from build123d import *

# Parameters (mm, degrees)
F0_W      = 1284.835703671
F0_H      = 12.4089680612
F1_DEPTH  = 571.5
F3_DEPTH  = 1143
F6_W      = 51.6073703766
F6_H      = 47.9507148266
F7_DEPTH  = 1778
F8_W      = 51.4650344849
F8_H      = 51.4650344849
F9_DEPTH  = 508
F10_W     = 63.6484324932
F10_H     = 50.9061813354
F10_W_2   = 66.0638809204
F10_H_2   = 51.4912605286
F11_DEPTH = 1092.2
F12_W     = 1241.9298887253
F12_H     = 1109.2171669006
F13_DEPTH = 139.7
F14_W     = 296.2205260992
F14_H     = 70.9949955344
F14_W_2   = 408.8332653046
F14_H_2   = 83.2355730236
F15_DEPTH = 1127.2688971291
F16_W     = 894.5828676224
F16_H     = 889.6675109863
F17_DEPTH = 1320.8


with BuildPart() as f1:
    # F0 (on Front) → F1 (new body, symmetric)
    with BuildSketch(Plane.XZ):
        with Locations((576.5165500343, -47.0742117614)):
            Rectangle(F0_W, F0_H)
    extrude(amount=F1_DEPTH, both=True)

    # F2 (on face) → F3 (join)
    with BuildSketch(Plane.XZ.offset(571.5)):
        Polygon((-65.9013018012, -53.278695792), (-65.9013018012, -40.8697277308), (-65.9013018012, 93.3853983879), (-249.7984468937, 93.3853983879), (-249.7984468937, 77.8451710939), (-80.1585838199, 77.8451710939), (-80.1585838199, -53.278695792), align=None)
    extrude(amount=-F3_DEPTH)

    # F5: F1 across plane


with BuildPart() as f1_1:
    add(f1.part)
    add(f1.part.mirror(Plane(origin=(569.387909025, 0, -17.3954870552), x_dir=(0, -1, 0), z_dir=(-1, 0, 0))))

    # F6 (on face) → F7 (join)
    with BuildSketch(Plane.XY.offset(-40.8697277308)):
        with Locations((569.3829655647, 546.9712764025)):
            Rectangle(F6_W, F6_H)
    extrude(amount=F7_DEPTH)

    # F8 (on mid) → F9 (join, symmetric)
    with BuildSketch(Plane(origin=(569.387909025, 0, 0), x_dir=(0, -1, 0), z_dir=(-1, 0, 0))):
        with Locations((-546.9267964363, 1710.9147310257)):
            Rectangle(F8_W, F8_H)
    extrude(amount=F9_DEPTH, both=True)

    # F10 (on face) → F11 (join)
    with BuildSketch(Plane.XZ.offset(-521.1942791939)):
        with Locations((93.3082550764, 1711.1941576004)):
            Rectangle(F10_W, F10_H)
        with Locations((1043.2767868042, 1710.7145786285)):
            Rectangle(F10_W_2, F10_H_2)
    extrude(amount=F11_DEPTH)

    # F12 (on face) → F13 (join)
    with BuildSketch(Plane.XY.offset(-40.8697277308)):
        with Locations((564.4726157188, 0)):
            Rectangle(F12_W, F12_H)
    extrude(amount=F13_DEPTH)

    # F14 (on face) → F15 (cut, through all)
    with BuildSketch(Plane.XZ.offset(554.6085834503)):
        with Locations((122.6859763265, 33.3608575165)):
            Rectangle(F14_W, F14_H)
        with Locations((898.7348079681, 28.4646395594)):
            Rectangle(F14_W_2, F14_H_2)
    extrude(amount=-F15_DEPTH, mode=Mode.SUBTRACT)

    # F16 (on face) → F17 (join)
    with BuildSketch(Plane.XY.offset(98.8302722692)):
        with Locations((564.4726157188, 0)):
            Rectangle(F16_W, F16_H)
    extrude(amount=F17_DEPTH)


solid = f1_1.part
CAD build for the part. Positions are in the model's coordinates, mm. A direction names the side the tool comes from. Coordinates: 2 decimals unless noted, no trailing zeros. Loops run counter-clockwise (first coordinate to the right, second up) from the corner with the lowest first, then second, coordinate; pieces in that order, holes last. Notation, with made-up numbers: (-30.75, 28.5) - (18.25, 28.5) arc R8 ccw to (18.25, 39.5) - close; hole circle Ø9 at (13.5, 49.25). An arc over 180 degrees is marked (long way). Write item = value, one per line. Start each with the question number.
Q1. Cut at A-A, the plane x = 9.5. List the corners of the cut face in (y, z).
Q2. Cut at C-C, the plane x = 218.5. List the corners of the cut face in (y, z).
Q3. Drill centre lines: L1, parallel to Z at x = 94, y = 389; L2, parallel to Z at x = 801, y = -14.5; L3, parallel to Z at x = 8, y = 45.5. Where is each one in solid material? Low to high.
Q4. Cut at B-B, the plane z = 1276.5. List the corners of the cut face in (x, y).
Q5. Which spindle directions (+Z, -Z, +X, -X, +Y, -Y) get a long thin tool onto all of the face, cutting with end or side? Do faces 1 (the flat face through (694.318, -8, 28)), 2 (the flat face through (1305, -8, 77.845)), 3 (the flat face through (1011.764, -6, 750)). Say none if no direction does.
Q6. Flat gauge pins, fed straight in: pin 1 Ø24 at (y, z) = (540, 1145) entering from -X; pin 2 Ø15.5 at (x, z) = (1046, 1698.5) entering from -Y; pin 3 Ø1 at (x, z) = (734.5, 402) entering from +Y. Where does each tip first touch, or does it go through?
Q7. Pull direction X, two halves, no side cores. Call faces 4 (the flat face through (115, 173, 1736.647)), 5 (the flat face through (-80.159, -8, 13)), 6 (the flat face through (1218.934, -8, 13)), 7 (the flat face through (896, -8, 70.082)): pulls with the +X half, pulls with the -X half, needs draft (parallel to the pull), parting line crosses it, or undercut.
Q8. Cut at D-D, the plane y = 218.5. Give the number of separate pieces and of enclosed holes in the cut face, then the cut area to 3 significant figures.
Computed:
q1.outline = (-571.5, -53.28) - (571.5, -53.28) - (571.5, -40.87) - (554.61, -40.87) - (554.61, -2.14) - (-554.61, -2.14) - (-554.61, -40.87) - (-571.5, -40.87) - close; (-554.61, 68.86) - (554.61, 68.86) - (554.61, 98.83) - (-554.61, 98.83) - close
q2.outline = (-571.5, -53.28) - (571.5, -53.28) - (571.5, -40.87) - (554.61, -40.87) - (554.61, -2.14) - (-554.61, -2.14) - (-554.61, -40.87) - (-571.5, -40.87) - close; (-554.61, 68.86) - (554.61, 68.86) - (554.61, 98.83) - (444.83, 98.83) - (444.83, 1419.63) - (-444.83, 1419.63) - (-444.83, 98.83) - (-554.61, 98.83) - close; (521.19, 1685.18) - (572.66, 1685.18) - (572.66, 1736.65) - (521.19, 1736.65) - close
q3.L1 = -53.28 to -2.14, 68.86 to 98.83, 1685.74 to 1736.65
q3.L2 = -53.28 to -13.15, 70.08 to 1419.63
q3.L3 = -53.28 to -2.14, 68.86 to 98.83
q4.outline = (117.18, -444.83) - (1011.76, -444.83) - (1011.76, 444.83) - (117.18, 444.83) - close; (543.58, 523) - (595.19, 523) - (595.19, 570.95) - (543.58, 570.95) - close
q5.face_1 = +Y, -Y
q5.face_2 = -Z, +X, +Y, -Y
q5.face_3 = +X, +Y, -Y
q6.pin_1 = 543.58
q6.pin_2 = -571.01
q6.pin_3 = 444.83
q7.face_4 = needs draft
q7.face_5 = pulls with the -X half
q7.face_6 = pulls with the +X half
q7.face_7 = undercut
q8.separate_pieces = 3
q8.enclosed_holes = 2
q8.area = 1,330,000 mm²
